The model under review builds one solid part; all positions refer to its coordinate system, in mm. A direction names the side the tool comes from. Round coordinates to 2 decimals unless told otherwise and drop trailing zeros. Write each loop counter-clockwise with the first axis right and the second up, starting at its lowest first coordinate (ties: lowest second). Pieces come first, ordered by that corner, then holes.
Item 1: Add section B-B (x = 4.9). Give the boundary of the cut face in (y, z).
Item 2: To check wall thickness, follow L1, parallel to Z at x = 26.55, y = -2.2; L2, parallel to X at y = -2.1, z = 8; L3, parallel to Y at x = 23.5, z = 8.5. State the ranges of each line that lie inside material, in increasing order.
Item 3: Draft analysis for pull direction Z (two halves, no side actions). For faces 1 (the face through (37.3, -27, 14)), 2 (the face through (36, -5, 0)), 3 (the face through (47.9, -5, 8)), state which applies: +Z half, -Z half, draft (parallel to the pull), parting line (faces both ways), or undercut.
Item 4: Machinability: for faces 4 (the face through (30.7, -6, 8)), 5 (the face through (18, -21.8, 14)), 6 (the face through (9, -11, 5)), which of the approach directions +Z, -Z, +X, -X, +Y, -Y give a long, thin tool a straight path to every point of the face, cutting with its end or side? Answer none if there is none.
Item 5: Clearance check with flat-ended pins moving along their axes: pin 1 Ø4 at (x, z) = (39.5, 5) entering from +Y; pin 2 Ø8 at (x, y) = (70.5, 16) entering from -Z; pin 3 Ø5.5 at (y, z) = (-6, 7) entering from +X; pin 4 Ø6 at (x, y) = (21, -27) entering from +Z. State where each tip first meets the part, or that it passes through.
Item 6: Add section A-A (z = 7.5). State how many separate pieces and enclosed holes the cut face has, plus the area to 3 significant figures.
Item 7: Add section D-D (x = 13.5). Give the boundary of the cut face in (y, z), plus the area to 3 significant figures.
Item 8: Add section C-C (y = 9). Give the boundary of the cut face in (x, z), plus the area to 3 significant figures.
```python
from build123d import *

# Parameters (mm, degrees)
ESQUISSE1_R                = 1.15
BOSS_EXTRU_1_DEPTH         = 16
ESQUISSE5_W                = 10
ESQUISSE5_H                = 4.5
ENL_V_MAT_EXTRU_3_DEPTH    = 12
ESQUISSE6_R                = 1.75
ENL_V_MAT_EXTRU_4_DEPTH    = 86.271756755
ESQUISSE12_W               = 7
ESQUISSE12_H               = 12
ENL_V_MAT_EXTRU_7_DEPTH    = 27
ESQUISSE14_W               = 23.3
ESQUISSE14_H               = 14.8
BOSS_EXTRU_2_DEPTH         = 4
CONG_1_R                   = 10
ESQUISSE15_R               = 6.25
ENL_V_MAT_EXTRU_8_DEPTH    = 18
CONG_2_R                   = 2
CONG_3_R                   = 7
R_P_TITION_LIN_AIRE1_COUNT = 2
R_P_TITION_LIN_AIRE1_PITCH = 25.5
ENL_V_MAT_EXTRU_9_DEPTH    = 40.213671452
ENL_V_START                = -4
ENL_V_MAT_EXTRU_10_DEPTH   = 88.47468181
R_P_TITION_LIN_AIRE2_COUNT = 2
R_P_TITION_LIN_AIRE2_PITCH = 25.5


with BuildPart() as part:
    # Esquisse1 → Boss.-Extru.1 (new body)
    with BuildSketch(Plane.XY):
        Polygon((0, 0), (67.35, 0), (67.35, 20), (77.35, 20), (77.35, -7), (37.3, -7), (37.3, -34), (30.3, -34), (30.3, -7), (7, -7), (7, -34), (0, -34), align=None)
        with Locations((4.9, -27.9)):
            Circle(ESQUISSE1_R, mode=Mode.SUBTRACT)
        with Locations((32.4, -27.9)):
            Circle(ESQUISSE1_R, mode=Mode.SUBTRACT)
    extrude(amount=BOSS_EXTRU_1_DEPTH)

    # Esquisse5 → Enlèv. mat.-Extru.3 (cut)
    with BuildSketch(Plane(origin=(0, 20, 0), x_dir=(1, 0, 0), z_dir=(0, 1, 0))):
        with Locations((72.35, -2.25)):
            Rectangle(ESQUISSE5_W, ESQUISSE5_H)
        with Locations((72.35, -13.75)):
            Rectangle(ESQUISSE5_W, ESQUISSE5_H)
    extrude(amount=-ENL_V_MAT_EXTRU_3_DEPTH, mode=Mode.SUBTRACT)

    # Esquisse6 → Enlèv. mat.-Extru.4 (cut, through all)
    with BuildSketch(Plane.XY.offset(11.5)):
        with Locations((72.35, 15)):
            Circle(ESQUISSE6_R)
        with BuildLine():
            Line((67.35, 15), (65.349467458, 15))
            Line((65.349467458, 15), (65.349467458, 22.000532542))
            Line((65.349467458, 22.000532542), (79.350532542, 22.000532542))
            Line((79.350532542, 22.000532542), (79.350532542, 15))
            Line((79.350532542, 15), (77.35, 15))
            ThreePointArc((77.35, 15), (72.35, 20), (67.35, 15))
        make_face()
    extrude(amount=-ENL_V_MAT_EXTRU_4_DEPTH, mode=Mode.SUBTRACT)

    # Esquisse12 → Enlèv. mat.-Extru.7 (cut)
    with BuildSketch(Plane(origin=(0, -34, 0), x_dir=(-1, 0, 0), z_dir=(0, -1, 0))):
        with Locations((-33.8, -6)):
            Rectangle(ESQUISSE12_W, ESQUISSE12_H)
    extrude(amount=-ENL_V_MAT_EXTRU_7_DEPTH, mode=Mode.SUBTRACT)

    # Esquisse14 → Boss.-Extru.2 (add)
    with BuildSketch(Plane.XY.offset(16)):
        with Locations((18.65, -14.4)):
            Rectangle(ESQUISSE14_W, ESQUISSE14_H)
    extrude(amount=-BOSS_EXTRU_2_DEPTH)

    # Congé1
    cong_1_edges = [part.edges().sort_by_distance(p)[0] for p in [
        (22.15, -7, 12),
        (7, -7, 6),
    ]]
    fillet(cong_1_edges, radius=CONG_1_R)

    # Esquisse15 → Enlèv. mat.-Extru.8 (cut)
    with BuildSketch(Plane.XY.offset(16)):
        with Locations((38.3, -13.25)):
            Circle(ESQUISSE15_R)
    extrude(amount=-ENL_V_MAT_EXTRU_8_DEPTH, mode=Mode.SUBTRACT)

    # Congé2
    cong_2_edges = [part.edges().sort_by_distance(p)[0] for p in [
        (37.3, -19.41948134, 14),
    ]]
    fillet(cong_2_edges, radius=CONG_2_R)

    # Congé3
    cong_3_edges = [part.edges().sort_by_distance(p)[0] for p in [
        (77.35, -7, 8),
    ]]
    fillet(cong_3_edges, radius=CONG_3_R)

    # Esquisse16 → Enlèvement de matière-Révolution1 (revolve, cut)
    with BuildSketch(Plane(origin=(0, 0, 8), x_dir=(-1, 0, 0), z_dir=(0, 0, -1)), mode=Mode.PRIVATE) as enl_vement_de_mati_re_r_volution1_sk:
        Polygon((-52.05, 0), (-52.05, -7), (-52.05, -57), (-48.05, -57), (-48.05, -7), (-49.55, -5.5), (-49.55, 0), align=None)
    enl_vement_de_mati_re_r_volution1 = revolve(enl_vement_de_mati_re_r_volution1_sk.sketch.rotate(Axis((52.05, 0, 8), (0, -1, 0)), 270), axis=Axis((52.05, 0, 8), (0, -1, 0)), mode=Mode.SUBTRACT)

    # Répétition linéaire1: Enlèvement de matière-Révolution1 ×2
    with Locations(*[(-i * R_P_TITION_LIN_AIRE1_PITCH, 0, 0) for i in range(1, R_P_TITION_LIN_AIRE1_COUNT)]):
        add(enl_vement_de_mati_re_r_volution1, mode=Mode.SUBTRACT)

    # Esquisse17 → Enlèv. mat.-Extru.9 (cut)
    with BuildSketch(Plane(origin=(77.35, 0, 0), x_dir=(0, 0, -1), z_dir=(1, 0, 0))):
        Polygon((-9, -7), (-16, -6), (-16, -7), align=None)
    extrude(amount=-ENL_V_MAT_EXTRU_9_DEPTH, mode=Mode.SUBTRACT)

    # Esquisse18 → Enlèv. mat.-Extru.10 (cut)
    with BuildSketch(Plane.XZ.offset(7).offset(ENL_V_START)):
        Polygon((56.2, 10.396003617), (56.2, 5.603996383), (52.05, 3.207992766), (47.9, 5.603996383), (47.9, 10.396003617), (52.05, 12.792007234), align=None)
    enl_v_mat_extru_10 = extrude(amount=ENL_V_MAT_EXTRU_10_DEPTH, mode=Mode.SUBTRACT)

    # Répétition linéaire2: Enlèv. mat.-Extru.10 ×2
    with Locations(*[(-i * R_P_TITION_LIN_AIRE2_PITCH, 0, 0) for i in range(1, R_P_TITION_LIN_AIRE2_COUNT)]):
        add(enl_v_mat_extru_10, mode=Mode.SUBTRACT)


solid = part.part
```
Numbers:
1. outline: (-34, 0) - (-29.05, 0) - (-29.05, 16) - (-34, 16) - close; (-26.75, 0) - (0, 0) - (0, 16) - (-26.75, 16) - close
2. L1: z = 0 to 5.5, 10.5 to 16
2. L2: x = 0 to 24.05, 29.05 to 49.55, 54.55 to 77.03
2. L3: y = -3 to 0
3. face 1: draft
3. face 2: -Z half
3. face 3: undercut
4. face 4: -Y
4. face 5: +Z, -Z, -Y
4. face 6: -Z, +X, -Y
5. pin 1: stops at y = 0
5. pin 2: stops at z = 4.5
5. pin 3: stops at x = 76.55
5. pin 4: passes through
6. separate pieces: 3
6. enclosed holes: 2
6. area: 844 mm2
7. outline: (-21.8, 12) - (-17, 12) arc R10 cw to (-7.63, 5.5) - (-7.63, 0) - (0, 0) - (0, 16) - (-21.8, 16) - close
7. area: 195 mm2
8. outline: (67.35, 4.5) - (77.35, 4.5) - (77.35, 11.5) - (67.35, 11.5) - close
8. area: 70.0 mm2
